Input: part model. Units: mm. Frame: model coordinates. Face numbers are marked on the shaded views. A direction names the side the tool comes from. Coordinates: 2 decimals unless noted, no trailing zeros. Write each loop counter-clockwise with the first axis right and the second up, starting at its lowest first coordinate (ties: lowest second). Pieces come first, ordered by that corner, then holes. Notation, with made-up numbers: (26, -27) - (41, -27) arc R14 ccw to (41, -23) - close; hole circle Ø5 at (-29, 19). An arc over 180 degrees is marked (long way). Use CSV: the item, a comma, the result in double quotes.
```python
from build123d import *

# Parameters (mm, degrees)
F0_R     = 13.1
F0_R_2   = 11.5
F1_DEPTH = 25
F0_R_3   = 19
F2_DEPTH = 2
F3_DEPTH = 23


with BuildPart() as f1:
    # F0 (on Top) → F1 (new body)
    with BuildSketch(Plane.XY):
        Circle(F0_R)
        Circle(F0_R_2, mode=Mode.SUBTRACT)
        Circle(F0_R_2)
    extrude(amount=F1_DEPTH)

    # F0 (on Top) → F2 (join)
    with BuildSketch(Plane.XY):
        Circle(F0_R_3)
        Circle(F0_R, mode=Mode.SUBTRACT)
    extrude(amount=F2_DEPTH)

    # F0 (on Top) → F3 (cut)
    with BuildSketch(Plane.XY):
        Circle(F0_R_2)
    extrude(amount=F3_DEPTH, mode=Mode.SUBTRACT)


solid = f1.part
```
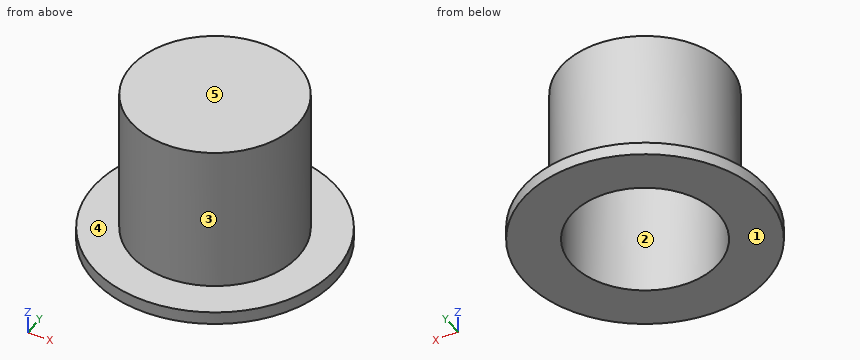
(1) Pin query (flat end, axial travel): pin 1 Ø2 at (y, z) = (10, 19) entering from +X; pin 2 Ø1 at (x, z) = (-11, 9.5) entering from -Y; pin 3 Ø8 at (x, y) = (13, -11.5) entering from +Z. Return the tip coordinate at first contact, or that it passes through.
Check values:
pin 1,"x = 9.52"
pin 2,"y = -7.83"
pin 3,"z = 2"
(2) Draft query along Y for the marked faces 1, 2 and 3. Return one class per face: pulls with the +Y half, pulls with the -Y half, needs draft (parallel to the pull), parting line crosses it, or undercut.
Check values:
face 1,"needs draft"
face 2,"undercut"
face 3,"parting line crosses it"
(3) Reachability of the marked faces 4 and 5 from +Z, -Z, +X, -X, +Y, -Y: full face, straight path, thin tool, end or side. Return the list, or none.
Check values:
face 4,"+Z"
face 5,"+Z, +X, -X, +Y, -Y"
(4) Ray query, probe 1 along Y at (x, z) = (0, 17.5); probe 2 along Z at (x, y) = (17, 0.5); probe 3 along X at (y, z) = (7, 17). Return the intervals inside material, ascending. Write a range as from..to.
Check values:
probe 1,"-13.1..-11.5, 11.5..13.1"
probe 2,"0..2"
probe 3,"-11.07..-9.12, 9.12..11.07"
(5) Cut plane D-D on x = -12.5. Return loops of the section in (y, z).
Check values:
outline,"(-14.31, 0) - (14.31, 0) - (14.31, 2) - (3.92, 2) - (3.92, 25) - (-3.92, 25) - (-3.92, 2) - (-14.31, 2) - close"
(6) Cut plane A-A on y = 0. Return loops of the section in (x, z).
Check values:
outline,"(-19, 0) - (-11.5, 0) - (-11.5, 23) - (11.5, 23) - (11.5, 0) - (19, 0) - (19, 2) - (13.1, 2) - (13.1, 25) - (-13.1, 25) - (-13.1, 2) - (-19, 2) - close"
(7) Cut plane C-C on z = 12.75. Return loops of the section in (x, y).
Check values:
outline,"circle Ø26.2 at (0, 0); hole circle Ø23 at (0, 0)"
